Source: three-view drawing plus pictorial views. Frame: mm from the lowest corner of the part. Give positions to 0.01 mm unless a question says otherwise; leave off trailing zeros. Write each loop counter-clockwise with the first axis right and the second up, starting at its lowest first coordinate (ties: lowest second). Pieces come first, ordered by that corner, then holes. Notation, with made-up numbers: (78.5, 53.5) -> (134.5, 53.5) arc R16 cw to (134.5, 79.5) -> close; hole circle Ø8 at (-32.5, 56.5). An arc over 180 degrees is marked (long way). Write item = value, one per line.
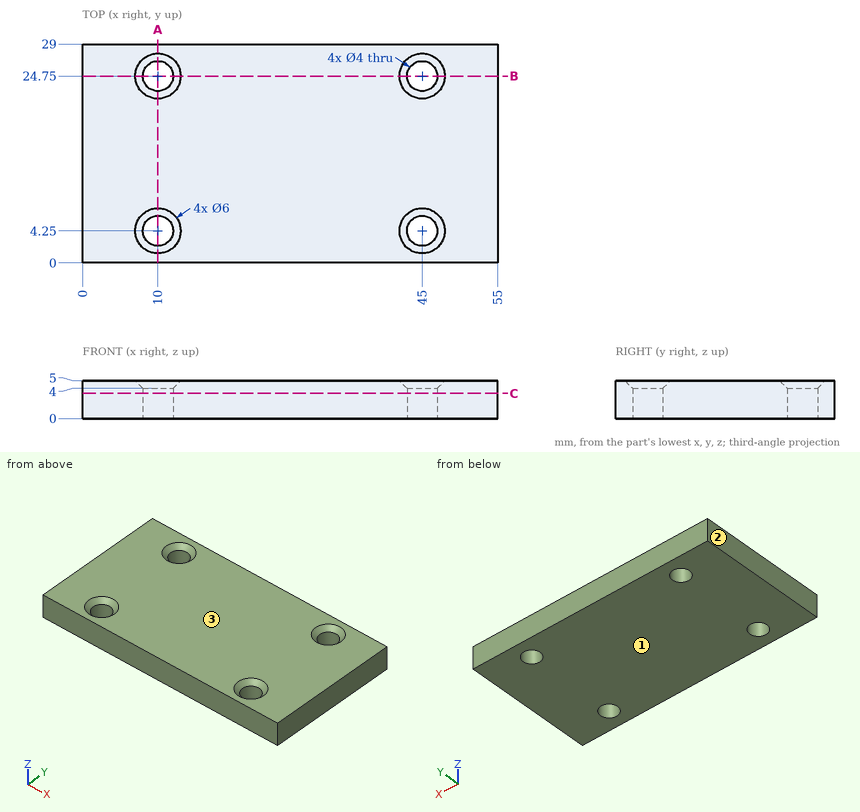
1) Cut plane B-B (y = 24.75). Return the cut outline in (x, z).
Computed:
outline = (0, 0) -> (8, 0) -> (8, 4) -> (7, 5) -> (0, 5) -> close; (12, 0) -> (43, 0) -> (43, 4) -> (42, 5) -> (13, 5) -> (12, 4) -> close; (47, 0) -> (55, 0) -> (55, 5) -> (48, 5) -> (47, 4) -> close
2) Contact query for a flat-ended pin moving along its axis: pin 1 (5 mm diameter, centred on x = 10, y = 4.25, fed in from +Z). Output: stop coordinate, or through.
Computed:
pin_1 = 4.5
3) Cut plane C-C (z = 3.35). Return the cut outline in (x, y).
Computed:
outline = (0, 0) -> (55, 0) -> (55, 29) -> (0, 29) -> close; hole circle Ø4 at (10, 4.25); hole circle Ø4 at (10, 24.75); hole circle Ø4 at (45, 4.25); hole circle Ø4 at (45, 24.75)
4) Material intervals for L1, parallel to Y at x = 10, z = 2.55; L2, parallel to X at y = 4.25, z = 3; L3, parallel to X at y = 6, z = 1.5, sorted ascending.
Computed:
L1 = 0 to 2.25, 6.25 to 22.75, 26.75 to 29
L2 = 0 to 8, 12 to 43, 47 to 55
L3 = 0 to 9.03, 10.97 to 44.03, 45.97 to 55
5) Draft query along Z for the marked faces 1, 2 and 3. Return one class per face: pulls with the +Z half, pulls with the -Z half, needs draft (parallel to the pull), parting line crosses it, or undercut.
Computed:
face_1 = pulls with the -Z half
face_2 = needs draft
face_3 = pulls with the +Z half
6) Cut plane A-A (x = 10). Return the cut outline in (y, z), then the cut area to 3 significant figures.
Computed:
outline = (0, 0) -> (2.25, 0) -> (2.25, 4) -> (1.25, 5) -> (0, 5) -> close; (6.25, 0) -> (22.75, 0) -> (22.75, 4) -> (21.75, 5) -> (7.25, 5) -> (6.25, 4) -> close; (26.75, 0) -> (29, 0) -> (29, 5) -> (27.75, 5) -> (26.75, 4) -> close
area = 103 mm²
